Source: CAD feature listing. Evaluate the final solid. Frame: model axes, mm. A direction names the side the tool comes from. Coordinates: 2 decimals unless noted, no trailing zeros. Loops run counter-clockwise (first coordinate to the right, second up) from the corner with the lowest first, then second, coordinate; pieces in that order, holes last. Notation, with made-up numbers: (-24.5, -28.5) -> (-0.5, -28.5) arc R16 ccw to (-0.5, -12.5) -> close; hole circle Ø8 at (-12.5, 37). An arc over 180 degrees is marked (long way). Answer as CSV lines item,"result".
Autodesk Fusion 360 part; units mm, degrees
sketch "Sketch1" plane through (0, 0, 0) normal (0, 1, 0) x (1, 0, 0)
  line L0 (0, 0) -> (40, 0)
  line L1 (34.9044, -14) -> (0, -14)
  line L2 (0, -14) -> (0, 0)
  line L3 (61.6428, -36.4361) -> (34.9044, -14)
  line L4 (70.6418, -25.7115) -> (61.6428, -36.4361)
  line L5 (40, 0) -> (70.6418, -25.7115)
  dimension "d1" = 40
  dimension "d2" = 14
  dimension "d3" = 14
  dimension "d4" = 40
  dimension "d5" = 140
extrude "Extrude1" add sketch "Sketch1" along normal blind 14
fillet "Fillet1" radius 2 10 edges at (17.4522, 0, 14) (20, 0, 0) (34.9044, 7, 14) (48.2736, 0, 25.2181) (17.4522, 14, 14) (55.3209, 0, 12.8558) (48.2736, 14, 25.2181) (55.3209, 14, 12.8558) (20, 14, 0) (40, 7, 0)
shell "Shell1" thickness 1 removed faces 2 at (0, 5.3333, 9.3333) at (66.7851, 5.3333, 30.3078)
sketch "Sketch2" plane through (0, 0, 0) normal (0, -1, 0) x (1, 0, 0)
  line L0 (39.2721, 2) -> (69.3562, 27.2436)
  line L1 (69.3562, 27.2436) -> (62.9283, 34.904)
  line L2 (62.9283, 34.904) -> (36.7476, 12.9358)
  arc A0 (34.1765, 12) -> (36.7476, 12.9358) centre (34.1765, 16) ccw
  line L3 (34.1765, 12) -> (0, 12)
  line L4 (0, 12) -> (0, 2)
  line L5 (0, 2) -> (39.2721, 2)
  circle A1 centre (0, 7) radius 9.5
  circle A2 centre (66.1423, 31.0738) radius 9.5
  dimension "d11" = 19
  dimension "d12" = 19
extrude "Extrude2" add sketch "Sketch2" along normal blind -16 and the other way blind -2 contours L0 L1 L2 A2 | L0 L1 L2 A2 | L3 L4 L5 A1 | L3 L4 L5 A1
sketch "Sketch3" plane through (0, -2, 0) normal (0, -1, 0) x (1, 0, 0)
  circle A0 centre (66.1423, 31.0738) radius 9.5
  circle A1 centre (66.1423, 31.0738) radius 7.5
  dimension "d17" = -2
extrude "Extrude3" cut sketch "Sketch3" against normal through all contours A1
sketch "Sketch4" plane through (0, -2, 0) normal (0, -1, 0) x (1, 0, 0)
  circle A0 centre (0, 7) radius 9.5
  line L0 (0, 7) -> (-5, 15.0777)
  circle A1 centre (0, 7) radius 7.5
  line L1 (0, 7) -> (-8.0777, 2)
  line L2 (0, 7) -> (0, 10.0999)
  line L3 (0, 10.0999) -> (0, 16.5)
  dimension "d19" = -2
  dimension "d20" = 90
  dimension "d21" = 5
extrude "Extrude4" cut sketch "Sketch4" against normal blind 40 contours A0 L0 A1 L1 | L0 A1 L2 L3 | A1 L1 L2 L3 | L0 A1 L1
(1) Pin query (flat end, axial travel): pin 1 Ø3 at (x, y) = (14, 10) entering from +Z; pin 2 Ø6 at (y, z) = (4, 20) entering from -X; pin 3 Ø2 at (x, z) = (46.5, 9.5) entering from +Y. Return the tip coordinate at first contact, or that it passes through.
Computed values:
pin 1,"z = 14"
pin 2,"x = 38.48"
pin 3,"y = 14"
(2) Cut plane A-A (x = 0). Return the cut outline in (y, z), then the cut area to 3 significant figures.
Computed values:
outline,"(-2, -2.5) -> (16, -2.5) -> (16, -0.5) -> (-2, -0.5) -> close; (-2, 14.5) -> (16, 14.5) -> (16, 16.5) -> (-2, 16.5) -> close"
area,"72.0 mm^2"
(3) Draft query along Y for faces 5 (the cylindrical face through (23.08, 13.4, 0.57)), 6 (the cylindrical face through (9.5, 6.9, 6.9)), 7 (the cylindrical face through (20.11, 0.57, 13.4)), 8 (the flat face through (-4.47, 6.87, 14.22)). Return one class per face: released by +Y, released by -Y, zero draft, split by the parting line, or undercut.
Computed values:
face 5,"released by +Y"
face 6,"undercut"
face 7,"released by -Y"
face 8,"zero draft"
(4) Cut plane C-C (z = 27.5). State how many separate pieces and enclosed holes the cut face has, then the cut area to 3 significant figures.
Computed values:
separate pieces,"2"
enclosed holes,"1"
area,"109 mm^2"
(5) Cut plane B-B (y = 8). Return the cut outline in (x, z).
Computed values:
outline,"(-8.08, 2) arc R9.5 ccw to (6.42, 0) -> (39.27, 0) arc R2 ccw to (40.56, 0.47) -> (65.72, 21.58) arc R9.5 ccw (long way) to (56.72, 32.31) -> (35.46, 14.47) arc R2 cw to (34.18, 14) -> (6.42, 14) arc R9.5 ccw to (-5, 15.08) -> (-3.95, 13.38) arc R7.5 cw (long way) to (-6.38, 3.05) -> close; hole (7.37, 1) -> (39.27, 1) arc R1 ccw to (39.91, 1.23) -> (64.36, 21.74) arc R9.5 cw to (56.64, 30.94) -> (36.1, 13.7) arc R3 cw to (34.18, 13) -> (7.37, 13) arc R9.5 cw to start; hole circle Ø15 at (66.14, 31.07)"
(6) Access query for faces 1 (the cylindrical face through (20.11, 13.4, 13.43)), 2 (the cylindrical face through (46.33, 0.57, 22.8)), 3 (the flat face through (20, 7, 14)), 4 (the cylindrical face through (35.216, 7.07, 13.186)). Directions: +Z, -Z, +X, -X, +Y, -Y. A direction counts if a zero-diameter tool reaches every point of the face in a straight line with its end or side. Return the directions, or none.
Computed values:
face 1,"+Z, +Y"
face 2,"+Z, -Y"
face 3,"+Z, +Y, -Y"
face 4,"none"
(7) Material intervals for L1, parallel to Z at x = 0, y = 3; L2, parallel to X at y = 5.5, z = 26; L3, parallel to Y at x = 40.5, z = 8, sorted ascending. Write a range as [from, to].
Computed values:
L1,"[-2.5, -0.5], [14.5, 16.5]"
L2,"[49.21, 50.76], [58.11, 60.62], [71.67, 74.17]"
L3,"[0, 1], [13, 14]"
